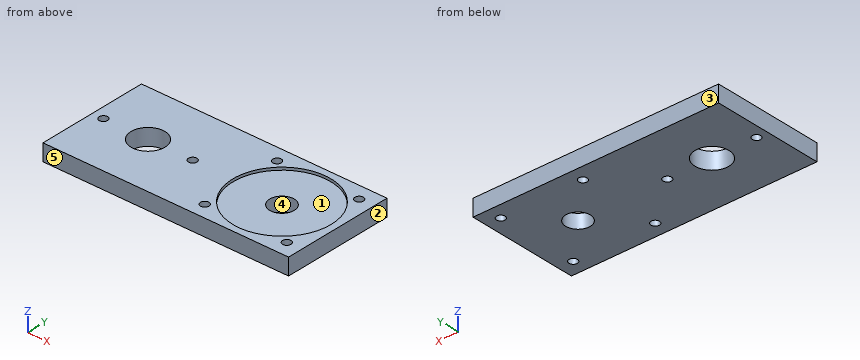
```python
from build123d import *

# Parameters (mm, degrees)
SKETCH1_W           = 152.4
SKETCH1_H           = 76.2
BOSS_EXTRUDE1_DEPTH = 9.525
SKETCH2_R           = 9.652
SKETCH2_R_2         = 6.985
SKETCH2_R_3         = 2.4003
CUT_EXTRUDE1_DEPTH  = 9.525
SKETCH3_R           = 27.94
CUT_EXTRUDE2_DEPTH  = 1.524
SKETCH4_W           = 152.4
SKETCH4_H           = 76.2
SKETCH4_W_2         = 139.7
SKETCH4_H_2         = 63.5
CUT_EXTRUDE3_DEPTH  = 10.525


with BuildPart() as part:
    # Sketch1 → Boss-Extrude1 (new body)
    with BuildSketch(Plane.XY):
        with Locations((76.2, 38.1)):
            Rectangle(SKETCH1_W, SKETCH1_H)
    extrude(amount=BOSS_EXTRUDE1_DEPTH)

    # Sketch2 → Cut-Extrude1 (cut)
    with BuildSketch(Plane.XY.offset(9.525)):
        with Locations((38.1, 38.1)):
            Circle(SKETCH2_R)
        with Locations((114.3, 38.1)):
            Circle(SKETCH2_R_2)
        with Locations((12.7, 38.1)):
            Circle(SKETCH2_R_3)
        with Locations((63.5, 38.1)):
            Circle(SKETCH2_R_3)
        with Locations((90.95994, 61.44006)):
            Circle(SKETCH2_R_3)
        with Locations((137.64006, 61.44006)):
            Circle(SKETCH2_R_3)
        with Locations((90.95994, 14.75994)):
            Circle(SKETCH2_R_3)
        with Locations((137.64006, 14.75994)):
            Circle(SKETCH2_R_3)
    extrude(amount=-CUT_EXTRUDE1_DEPTH, mode=Mode.SUBTRACT)

    # Sketch3 → Cut-Extrude2 (cut)
    with BuildSketch(Plane.XY.offset(9.525)):
        with Locations((114.3, 38.1)):
            Circle(SKETCH3_R)
    extrude(amount=-CUT_EXTRUDE2_DEPTH, mode=Mode.SUBTRACT)

    # Sketch4 → Cut-Extrude3 (cut, through all)
    with BuildSketch(Plane(origin=(0, 0, 0), x_dir=(-1, 0, 0), z_dir=(0, 0, -1))):
        with Locations((-76.2, 38.1)):
            Rectangle(SKETCH4_W, SKETCH4_H)
        with Locations((-76.2, 38.1)):
            Rectangle(SKETCH4_W_2, SKETCH4_H_2, mode=Mode.SUBTRACT)
    extrude(amount=-CUT_EXTRUDE3_DEPTH, mode=Mode.SUBTRACT)


solid = part.part
```
Verification items for the finished model (mm, model axes). Face numbers are marked on the shaded views. A direction names the side the tool comes from. Coordinates: 2 decimals unless noted, no trailing zeros. Order: outer loops, then holes, each group sorted by start corner. A loop starts at its lowest first (then second) coordinate and runs counter-clockwise, first axis right, second up. Notation, with made-up numbers: (39.5, 22) -> (95.5, 22) arc R33 cw to (95.5, 53) -> close; hole circle Ø8 at (35.5, 9.5). An arc over 180 degrees is marked (long way). Put each result on its own line as item: value. Start each with the question number.
1) Material ranges on L1, parallel to Y at x = 38.1, z = 7; L2, parallel to Y at x = 114.3, z = 6 (3 decimals); L3, parallel to Z at x = 133, y = 21, recorded low to high.
2) Tool access check on the marked faces 1 and 2. Record the directions out of +Z, -Z, +X, -X, +Y, -Y that give a thin tool (end or side, any length) a straight path to the whole face; none if there is none.
3) Cross-section at A-A (x = 12.7). Enter the section's corners in (y, z) (3 decimals).
4) Cross-section at D-D (z = 2.5). State how many separate pieces and enclosed holes the cut face has, plus the area to 3 significant figures.
5) Cross-section at B-B (x = 114.3). Enter the section's corners in (y, z) (3 decimals), plus the area to 3 significant figures.
6) Release check for a two-part mould opening along Y. For the marked faces 3, 4 and 5 record: pulls with the +Y half, pulls with the -Y half, needs draft (parallel to the pull), parting line crosses it, or undercut.
7) Go/stop test with flat-tipped pins: pin 1 (18 mm diameter, centred on x = 114.3, y = 38.1, fed in from +Z); pin 2 (4 mm diameter, centred on x = 12.7, y = 38.1, fed in from +Z). Record where each tip stops, or that it passes through.
Geometry check:
1. L1: y = 6.35 to 28.45, 47.75 to 69.85
1. L2: y = 6.35 to 31.115, 45.085 to 69.85
1. L3: z = 0 to 8
2. face 1: +Z
2. face 2: +Z, -Z, +X, +Y, -Y
3. outline: (6.35, 0) -> (35.7, 0) -> (35.7, 9.525) -> (6.35, 9.525) -> close; (40.5, 0) -> (69.85, 0) -> (69.85, 9.525) -> (40.5, 9.525) -> close
4. separate pieces: 1
4. enclosed holes: 8
4. area: 8,320 mm^2
5. outline: (6.35, 0) -> (31.115, 0) -> (31.115, 8.001) -> (10.16, 8.001) -> (10.16, 9.525) -> (6.35, 9.525) -> close; (45.085, 0) -> (69.85, 0) -> (69.85, 9.525) -> (66.04, 9.525) -> (66.04, 8.001) -> (45.085, 8.001) -> close
5. area: 408 mm^2
6. face 3: pulls with the +Y half
6. face 4: undercut
6. face 5: pulls with the -Y half
7. pin 1: stops at z = 8
7. pin 2: passes through
